Verification items for this drawing (mm, ordinates from the low corner). Coordinates: 2 decimals unless noted, no trailing zeros. Order: outer loops, then holes, each group sorted by start corner. A loop starts at its lowest first (then second) coordinate and runs counter-clockwise, first axis right, second up. Notation, with made-up numbers: (4.25, -18.75) -> (34.25, -18.75) arc R21 ccw to (34.25, 1.25) -> close; hole circle Ø8 at (47.25, 78.5). An arc over 180 degrees is marked (long way). Put each result on its own line as item: value. Start each with the question number.
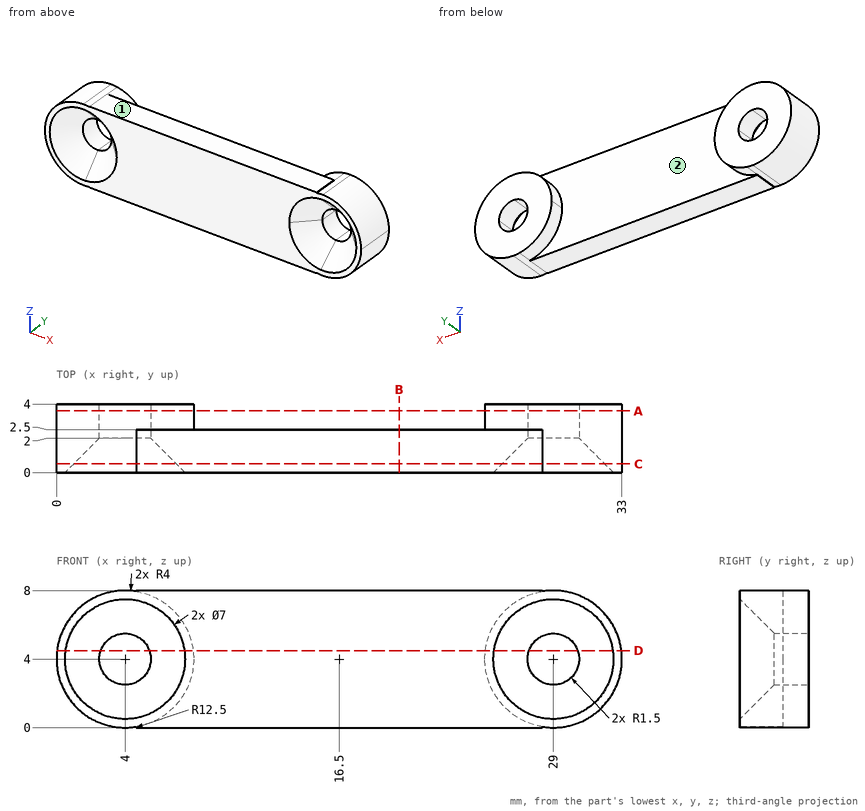
1) Sectioned sample at A-A (y = 3.6). Record the boundary of the cut face in (x, z), plus the area to 3 significant figures.
2) Sectioned sample at B-B (x = 20). Record the boundary of the cut face in (y, z), plus the area to 3 significant figures.
3) Mould release check, pull along X, two halves, no side actions. Record for the marked faces 1 and 2: +X half, -X half, draft (parallel to the pull), parting line (faces both ways), or undercut.
4) Sectioned sample at C-C (y = 0.5). Record the boundary of the cut face in (x, z), plus the area to 3 significant figures.
5) Scan lines: line 1 along X through (y, z) = (2.8, 2.75); line 2 along X through (y, z) = (0.9, 5.75); line 3 along X through (y, z) = (2.85, 3.75). Record each from-to range of solid material in increasing order. Write a range as [from, to].
6) Gauge pin test, flat ends, axial feed: pin 1 (2.5 mm diameter, centred on x = 16, z = 4, fed in from +Y); pin 2 (4 mm diameter, centred on x = 18, z = 6, fed in from -Y); pin 3 (1.5 mm diameter, centred on y = 1.5, z = 6, fed in from -X). Record the tip position at first contact, or that the pin passes through.
7) Sectioned sample at D-D (z = 4.5). State how many separate pieces and enclosed holes the cut face has, plus the area to 3 significant figures.
Entries:
1. outline: circle Ø8 at (4, 4); circle Ø8 at (29, 4); hole circle Ø3 at (4, 4); hole circle Ø3 at (29, 4)
1. area: 86.4 mm2
2. outline: (0, 0) -> (2.5, 0) -> (2.5, 8) -> (0, 8) -> close
2. area: 20.0 mm2
3. face 1: draft
3. face 2: undercut
4. outline: (4.64, 0.05) arc R12.5 ccw to (4.66, 0) -> (28.34, 0) arc R12.5 ccw to (28.36, 0.05) arc R4 ccw (long way) to (28.36, 7.95) arc R12.5 ccw to (28.34, 8) -> (4.66, 8) arc R12.5 ccw to (4.64, 7.95) arc R4 ccw (long way) to start; hole circle Ø6 at (4, 4); hole circle Ø6 at (29, 4)
4. area: 194 mm2
5. line 1: x = [0.2, 3.17], [4.83, 7.8], [25.2, 28.17], [29.83, 32.8]
5. line 2: x = [0.4, 2.08], [5.92, 27.08], [30.92, 32.6]
5. line 3: x = [0.01, 2.52], [5.48, 7.99], [25.01, 27.52], [30.48, 32.99]
6. pin 1: stops at y = 2.5
6. pin 2: stops at y = 0
6. pin 3: stops at x = 0.2
7. separate pieces: 3
7. enclosed holes: 0
7. area: 75.3 mm2
